Part print with two shaded views. Sizes in mm from the minimum x, y, z corner. A direction names the side the tool comes from. Round coordinates to 2 decimals unless told otherwise and drop trailing zeros. Loops run counter-clockwise (first coordinate to the right, second up) from the corner with the lowest first, then second, coordinate; pieces in that order, holes last.
(1) Cut at D-D on x = 6.25. List the corners of the cut face in (y, z) (1 decimal), then the cut area to 3 significant figures.
(2) Flat gauge pins, fed straight in: pin 1 (5 mm diameter, centred on x = 12, y = 13, fed in from -Z); pin 2 (6 mm diameter, centred on y = 3, z = 2.5, fed in from -X) (1 decimal); pin 3 (1 mm diameter, centred on x = 11.5, y = 13.5, fed in from -Z) (1 decimal); pin 4 (1.7 mm diameter, centred on y = 12, z = 6.5, fed in from -X). Where does each tip first touch, or does it go through?
(3) Tool access for the marked faces 4 and 5: list every direction of +Z, -Z, +X, -X, +Y, -Y with a clear straight run to the whole face (end or side of a thin tool).
(4) Mould opens along X. For the marked faces 1, 2 and 3 say: +X half, -X half, draft (parallel to the pull), parting line (faces both ways), or undercut.
(5) Cut at A-A on y = 8. List the corners of the cut face in (x, z) (1 decimal), then the cut area to 3 significant figures.
(6) Cut at C-C on y = 1.25. List the corners of the cut face in (x, z).
(7) Cut at B-B on z = 7.5. List the corners of the cut face in (x, y), then the cut area to 3 significant figures.
(8) Probe probe 1 along Z at (x, y) = (5, 12.5) (1 decimal); probe 2 along Z at (x, y) = (9, 12) (1 decimal); probe 3 along X at (y, z) = (11, 7.25) (1 decimal). List the from-to ranges inside material, lowest first.
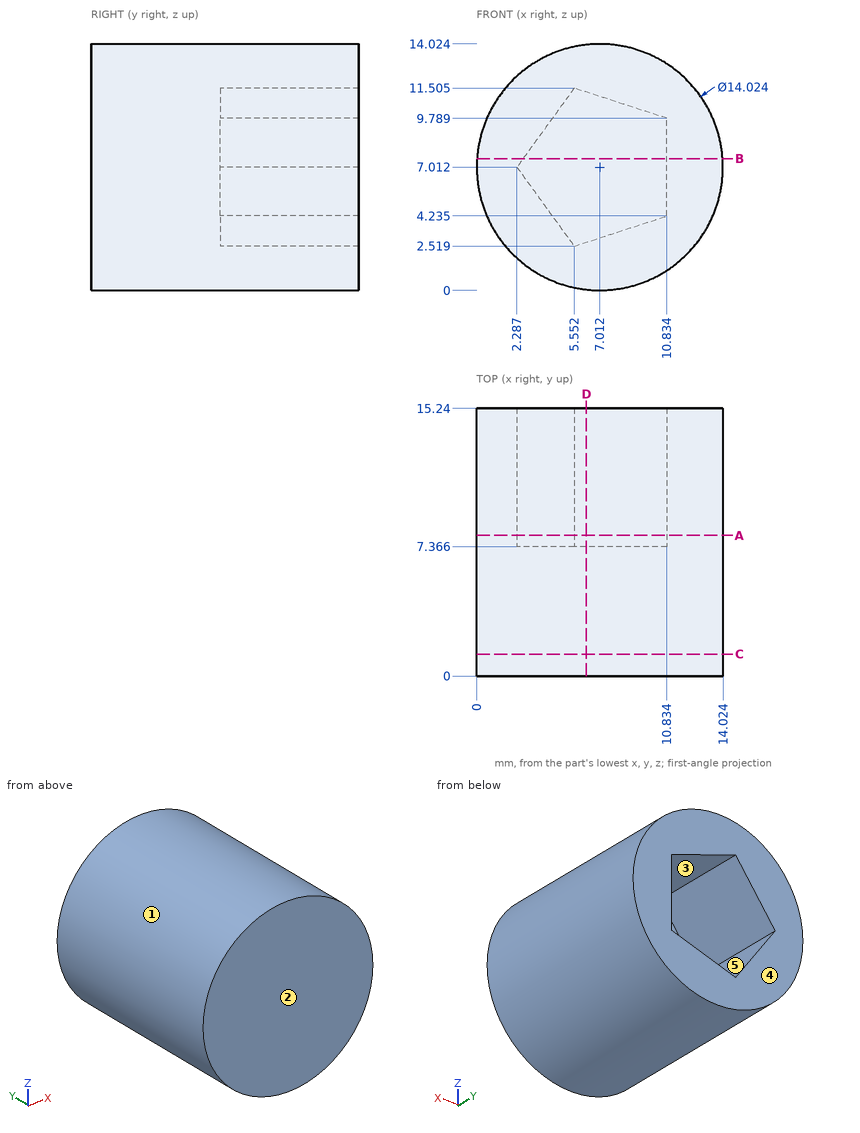
Final values:
1. outline: (0, 0) - (15.2, 0) - (15.2, 2.7) - (7.4, 2.7) - (7.4, 11.3) - (15.2, 11.3) - (15.2, 14) - (0, 14) - close
1. area: 145 mm2
2. pin 1: stops at z = 0.46
2. pin 2: stops at x = 0.2
2. pin 3: stops at z = 1.2
2. pin 4: stops at x = 0
3. face 4: +Z, -Z, +X, -X, +Y
3. face 5: +Y
4. face 1: parting line
4. face 2: draft
4. face 3: undercut
5. outline: circle Ø14 at (7, 7); hole (2.3, 7) - (5.6, 2.5) - (10.8, 4.2) - (10.8, 9.8) - (5.6, 11.5) - close
5. area: 101 mm2
6. outline: circle Ø14.02 at (7.01, 7.01)
7. outline: (0.02, 0) - (14.01, 0) - (14.01, 15.24) - (10.83, 15.24) - (10.83, 7.37) - (2.64, 7.37) - (2.64, 15.24) - (0.02, 15.24) - close
7. area: 149 mm2
8. probe 1: z = 0.3 to 3.3, 10.7 to 13.7
8. probe 2: z = 0.3 to 3.6, 10.4 to 13.7
8. probe 3: x = 0 to 2.5, 10.8 to 14
